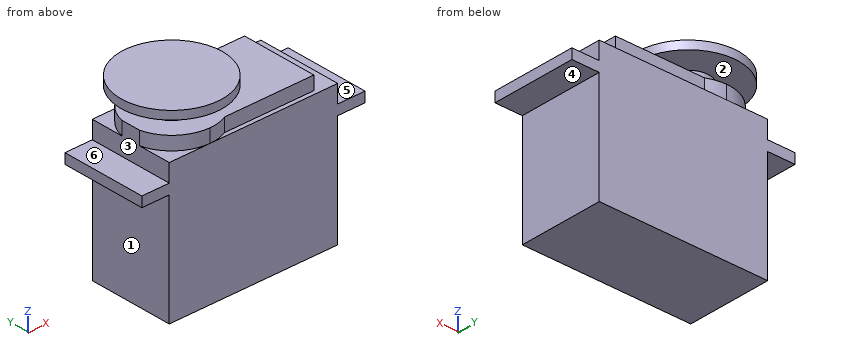
```python
from build123d import *

# Parameters (mm, degrees)
SKETCH1_W           = 40
SKETCH1_H           = 20
BOSS_EXTRUDE1_DEPTH = 33
SKETCH3_W           = 2.4
SKETCH3_H           = 20
BOSS_EXTRUDE2_DEPTH = 6.5
SKETCH3_2_W         = 2.4
SKETCH3_2_H         = 20
BOSS_EXTRUDE3_DEPTH = 46.5
SKETCH4_R           = 5
BOSS_EXTRUDE4_DEPTH = 7.5
SKETCH5_R           = 12
BOSS_EXTRUDE5_DEPTH = 2
SKETCH6_R           = 5
BOSS_EXTRUDE6_DEPTH = 3.2


with BuildPart() as part:
    # Sketch1 → Boss-Extrude1 (new body)
    with BuildSketch(Plane.XY):
        with Locations((20, 10)):
            Rectangle(SKETCH1_W, SKETCH1_H)
    extrude(amount=BOSS_EXTRUDE1_DEPTH)

    # Sketch3 → Boss-Extrude2 (add)
    with BuildSketch(Plane(origin=(40, 0, 0), x_dir=(0, 0, -1), z_dir=(1, 0, 0))):
        with Locations((-27.6, 10)):
            Rectangle(SKETCH3_W, SKETCH3_H)
    extrude(amount=BOSS_EXTRUDE2_DEPTH)

    # Sketch3_2 → Boss-Extrude3 (add)
    with BuildSketch(Plane(origin=(40, 0, 0), x_dir=(0, 0, -1), z_dir=(1, 0, 0))):
        with Locations((-27.6, 10)):
            Rectangle(SKETCH3_2_W, SKETCH3_2_H)
    extrude(amount=-BOSS_EXTRUDE3_DEPTH)

    # Sketch4 → Boss-Extrude4 (add)
    with BuildSketch(Plane.XY.offset(33)):
        with Locations(Location((9.726417673, 10, 0), (0, 0, 180))):
            Circle(SKETCH4_R)
    extrude(amount=BOSS_EXTRUDE4_DEPTH)

    # Sketch5 → Boss-Extrude5 (add)
    with BuildSketch(Plane.XY.offset(40.5)):
        with Locations((9.726417673, 10)):
            Circle(SKETCH5_R)
    extrude(amount=BOSS_EXTRUDE5_DEPTH)

    # Sketch6 → Boss-Extrude6 (add)
    with BuildSketch(Plane.XY.offset(33)):
        with BuildLine():
            Line((35.25, 1), (35.25, 19))
            Line((35.25, 19), (14.085316617, 19))
            ThreePointArc((14.085316617, 19), (11.962485651, 19.746794345), (9.726417673, 20))
            ThreePointArc((9.726417673, 20), (3.530895586, 17.849554514), (0, 12.323101213))
            Line((0, 12.323101213), (0, 7.676898787))
            ThreePointArc((0, 7.676898787), (3.530895586, 2.150445486), (9.726417673, 0))
            ThreePointArc((9.726417673, 0), (11.962485651, 0.253205655), (14.085316617, 1))
            Line((14.085316617, 1), (35.25, 1))
        make_face()
        with Locations((9.726417673, 10)):
            Circle(SKETCH6_R, mode=Mode.SUBTRACT)
    extrude(amount=BOSS_EXTRUDE6_DEPTH)


solid = part.part
```
Part model, mm, in its own coordinate system. Face numbers are marked on the shaded views. A direction names the side the tool comes from. Round coordinates to 2 decimals unless told otherwise and drop trailing zeros. Loops run counter-clockwise (first coordinate to the right, second up) from the corner with the lowest first, then second, coordinate; pieces in that order, holes last.
Item 1: Drop flat-ended pins along their axis: P1, Ø3.5, axis at y = 8, z = 31, coming from the +X side; P2, Ø16.5, axis at x = 17, z = 19.5, coming from the -Y side; P3, Ø3, axis at x = -2.5, y = 9.5, coming from the -Z side; P4, Ø12, axis at x = 13.5, y = 15.5, coming from the -Z side. Give the stop position or say it passes through.
Item 2: Cut at D-D, the plane x = 42.5. Give the cut face in (y, z), then the cut area to 3 significant figures.
Item 3: Cut at A-A, the plane y = 1.75. Give the cut face in (x, z).
Item 4: 3-axis set-ups, long thin cutter, end or side, ignore diameter. For the marked faces 1, 2 and 3: which of +Z, -Z, +X, -X, +Y, -Y reach the whole face in a straight line?
Item 5: Cut at B-B, the plane y = 10. Give the cut face in (x, z).
Item 6: Cut at C-C, the plane x = 16. Give the cut face in (y, z).
Item 7: Drill centre lines: line 1 (Z direction, x = 11, y = 3); line 2 (Y direction, x = 8, z = 15); line 3 (X direction, y = 15.75, z = 31.5). Where is each one in solid material? Low to high.
Item 8: Mould opens along Z. For the marked faces 4, 5 and 6 say: +Z half, -Z half, draft (parallel to the pull), parting line (faces both ways), or undercut.
A:
1. P1: stops at x = 40
1. P2: stops at y = 0
1. P3: stops at z = 26.4
1. P4: stops at z = 0
2. outline: (0, 26.4) - (20, 26.4) - (20, 28.8) - (0, 28.8) - close
2. area: 48.0 mm2
3. outline: (-6.5, 26.4) - (0, 26.4) - (0, 0) - (40, 0) - (40, 26.4) - (46.5, 26.4) - (46.5, 28.8) - (40, 28.8) - (40, 33) - (35.25, 33) - (35.25, 36.2) - (4.08, 36.2) - (4.08, 33) - (0, 33) - (0, 28.8) - (-6.5, 28.8) - close; (1.01, 40.5) - (18.44, 40.5) - (18.44, 42.5) - (1.01, 42.5) - close
4. face 1: -Z, -X, +Y, -Y
4. face 2: none
4. face 3: -X, +Y, -Y
5. outline: (-6.5, 26.4) - (0, 26.4) - (0, 0) - (40, 0) - (40, 26.4) - (46.5, 26.4) - (46.5, 28.8) - (40, 28.8) - (40, 33) - (35.25, 33) - (35.25, 36.2) - (14.73, 36.2) - (14.73, 40.5) - (21.73, 40.5) - (21.73, 42.5) - (-2.27, 42.5) - (-2.27, 40.5) - (4.73, 40.5) - (4.73, 36.2) - (0, 36.2) - (0, 28.8) - (-6.5, 28.8) - close
6. outline: (-0.23, 40.5) - (20.23, 40.5) - (20.23, 42.5) - (-0.23, 42.5) - close; (0, 0) - (20, 0) - (20, 33) - (19, 33) - (19, 36.2) - (1, 36.2) - (1, 33) - (0, 33) - close
7. line 1: z = 0 to 36.2, 40.5 to 42.5
7. line 2: y = 0 to 20
7. line 3: x = 0 to 40
8. face 4: -Z half
8. face 5: +Z half
8. face 6: undercut
